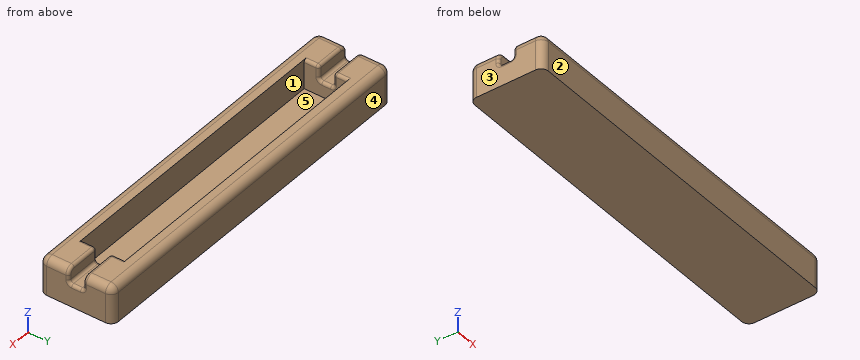
from build123d import *

# Parameters (mm, degrees)
F0_W         = 25
F0_H         = 5
F1_DEPTH     = 2.5
F2_W         = 20
F2_H         = 3
F3_DEPTH     = 2
F4_W         = 2.5
F4_H         = 1
F5_DEPTH     = 1
F6_F1_R      = 0.2
F6_F2_R      = 0.2
F7_T1_DEPTH  = 24
F7_T3_DEPTH  = 1.5
F7_T5_DEPTH  = 3.25
F7_T7_DEPTH  = 1.5
F7_T10_ANGLE = 90
F7_T12_ANGLE = 90
F7_T14_ANGLE = 90
F7_T16_ANGLE = 90
F7_S19_W     = 0.5
F7_S19_H     = 0.5
F7_T20_DEPTH = 0.5
F7_S25_W     = 0.5
F7_S25_H     = 0.5
F7_T26_DEPTH = 0.5
F7_S31_W     = 0.5
F7_S31_H     = 0.5
F7_T32_DEPTH = 0.5
F7_S37_W     = 0.5
F7_S37_H     = 0.5
F7_T38_DEPTH = 0.5


# Not quite as in the source:
# - a fillet or chamfer that OpenCascade refuses, or shapes differently, is made with other operations: its cross-section is extruded or revolved along the edge and cut away or added


with BuildPart() as f1:
    # F0 (on Top) → F1 (new body)
    with BuildSketch(Plane.XY):
        Rectangle(F0_W, F0_H)
    extrude(amount=F1_DEPTH)

    # F2 (on face) → F3 (cut)
    with BuildSketch(Plane.XY.offset(2.5)):
        Rectangle(F2_W, F2_H)
    extrude(amount=-F3_DEPTH, mode=Mode.SUBTRACT)

    # F4 (on face) → F5 (cut)
    with BuildSketch(Plane.XY.offset(2.5)):
        with Locations((-11.25, 0)):
            Rectangle(F4_W, F4_H)
        with Locations((11.25, 0)):
            Rectangle(F4_W, F4_H)
    extrude(amount=-F5_DEPTH, mode=Mode.SUBTRACT)

    # F6: fillet of radius 0.2 on 16 edges, made by hand

    # F6_f1
    f6_f1_edges = [f1.edges().sort_by_distance(p)[0] for p in [
        (-11.25, -0.5, 1.5),
        (-11.25, 0.5, 1.5),
        (11.25, -0.5, 1.5),
        (11.25, 0.5, 1.5),
    ]]
    fillet(f6_f1_edges, radius=F6_F1_R)

    # F6_f2
    f6_f2_edges = [f1.edges().sort_by_distance(p)[0] for p in [
        (-10, -0.5, 2.1),
        (10, 0, 1.5),
        (12.5, -0.5, 2.1),
        (-12.5, 0.5, 2.1),
        (-11.25, 0.5, 2.5),
        (-11.25, -0.5, 2.5),
        (11.25, 0.5, 2.5),
        (11.25, -0.5, 2.5),
        (-10, 1, 2.5),
        (10, 1, 2.5),
        (10, -1, 2.5),
        (-10, -1, 2.5),
        (-12.5, 0.4414213562, 1.5585786438),
        (12.5, -0.4414213562, 1.5585786438),
        (10, 0.4414213562, 1.5585786438),
        (10, -0.4414213562, 1.5585786438),
        (-10, -0.4414213562, 1.5585786438),
    ]]
    fillet(f6_f2_edges, radius=F6_F2_R)

    # F7: fillet of radius 0.5 on 10 edges, made by hand

    # F7_s2 → F7_t1 (cut)
    with BuildSketch(Plane.YZ.offset(-12)):
        with BuildLine():
            ThreePointArc((-2.5, 2), (-2.3535533906, 2.3535533906), (-2, 2.5))
            Line((-2, 2.5), (-2.5, 2.5))
            Line((-2.5, 2.5), (-2.5, 2))
        make_face()
        with BuildLine():
            ThreePointArc((2, 2.5), (2.3535533906, 2.3535533906), (2.5, 2))
            Line((2.5, 2), (2.5, 2.5))
            Line((2.5, 2.5), (2, 2.5))
        make_face()
    extrude(amount=F7_T1_DEPTH, mode=Mode.SUBTRACT)

    # F7_s4 → F7_t3 (cut)
    with BuildSketch(Plane.XZ.offset(0.5)):
        with BuildLine():
            ThreePointArc((-12, 2.5), (-12.3535533906, 2.3535533906), (-12.5, 2))
            Line((-12.5, 2), (-12.5, 2.5))
            Line((-12.5, 2.5), (-12, 2.5))
        make_face()
        with BuildLine():
            ThreePointArc((12.5, 2), (12.3535533906, 2.3535533906), (12, 2.5))
            Line((12, 2.5), (12.5, 2.5))
            Line((12.5, 2.5), (12.5, 2))
        make_face()
    extrude(amount=F7_T3_DEPTH, mode=Mode.SUBTRACT)

    # F7_s6 → F7_t5 (cut)
    with BuildSketch(Plane.XY.offset(-1.25)):
        with BuildLine():
            ThreePointArc((-12, -2.5), (-12.3535533906, -2.3535533906), (-12.5, -2))
            Line((-12.5, -2), (-12.5, -2.5))
            Line((-12.5, -2.5), (-12, -2.5))
        make_face()
        with BuildLine():
            ThreePointArc((12.5, -2), (12.3535533906, -2.3535533906), (12, -2.5))
            Line((12, -2.5), (12.5, -2.5))
            Line((12.5, -2.5), (12.5, -2))
        make_face()
        with BuildLine():
            ThreePointArc((-12, 2.5), (-12.3535533906, 2.3535533906), (-12.5, 2))
            Line((-12.5, 2), (-12.5, 2.5))
            Line((-12.5, 2.5), (-12, 2.5))
        make_face()
        with BuildLine():
            ThreePointArc((12.5, 2), (12.3535533906, 2.3535533906), (12, 2.5))
            Line((12, 2.5), (12.5, 2.5))
            Line((12.5, 2.5), (12.5, 2))
        make_face()
    extrude(amount=F7_T5_DEPTH, mode=Mode.SUBTRACT)

    # F7_s8 → F7_t7 (cut)
    with BuildSketch(Plane.XZ.offset(-2)):
        with BuildLine():
            ThreePointArc((-12, 2.5), (-12.3535533906, 2.3535533906), (-12.5, 2))
            Line((-12.5, 2), (-12.5, 2.5))
            Line((-12.5, 2.5), (-12, 2.5))
        make_face()
        with BuildLine():
            ThreePointArc((12.5, 2), (12.3535533906, 2.3535533906), (12, 2.5))
            Line((12, 2.5), (12.5, 2.5))
            Line((12.5, 2.5), (12.5, 2))
        make_face()
    extrude(amount=F7_T7_DEPTH, mode=Mode.SUBTRACT)

    # F7_s9 → F7_t10 (revolve, cut)
    with BuildSketch(Plane.XY.offset(2)):
        with BuildLine():
            ThreePointArc((12.3, 0.5), (12.4414213562, 0.5585786438), (12.5, 0.7))
            Line((12.5, 0.7), (12.5, 0.5))
            Line((12.5, 0.5), (12.3, 0.5))
        make_face()
    revolve(axis=Axis((12, 0.5, 2), (0, -1, 0)), revolution_arc=F7_T10_ANGLE, mode=Mode.SUBTRACT)

    # F7_s11 → F7_t12 (revolve, cut)
    with BuildSketch(Plane.YZ.offset(-12)):
        with BuildLine():
            ThreePointArc((0.5, 2.3), (0.5585786438, 2.4414213562), (0.7, 2.5))
            Line((0.7, 2.5), (0.5, 2.5))
            Line((0.5, 2.5), (0.5, 2.3))
        make_face()
    revolve(axis=Axis((-12, 0.5, 2), (0, -1, 0)), revolution_arc=F7_T12_ANGLE, mode=Mode.SUBTRACT)

    # F7_s13 → F7_t14 (revolve, cut)
    with BuildSketch(Plane.YZ.offset(12)):
        with BuildLine():
            ThreePointArc((-0.5, 2.3), (-0.5585786438, 2.4414213562), (-0.7, 2.5))
            Line((-0.7, 2.5), (-0.5, 2.5))
            Line((-0.5, 2.5), (-0.5, 2.3))
        make_face()
    revolve(axis=Axis((12, -0.5, 2), (0, 1, 0)), revolution_arc=F7_T14_ANGLE, mode=Mode.SUBTRACT)

    # F7_s15 → F7_t16 (revolve, cut)
    with BuildSketch(Plane.XY.offset(2)):
        with BuildLine():
            ThreePointArc((-12.3, -0.5), (-12.4414213562, -0.5585786438), (-12.5, -0.7))
            Line((-12.5, -0.7), (-12.5, -0.5))
            Line((-12.5, -0.5), (-12.3, -0.5))
        make_face()
    revolve(axis=Axis((-12, -0.5, 2), (0, 1, 0)), revolution_arc=F7_T16_ANGLE, mode=Mode.SUBTRACT)


with BuildPart() as f7_tool18:
    # F7_s19 → F7_t20 (new body)
    with BuildSketch(Plane.XY.offset(2)):
        with Locations((-12.25, -2.25)):
            Rectangle(F7_S19_W, F7_S19_H)
    extrude(amount=F7_T20_DEPTH)

    # F7_s21 → F7_t22 (revolve, cut)
    with BuildSketch(Plane(origin=(-12, -2, 2), x_dir=(0.7071067812, 0.7071067812, 0), z_dir=(0.7071067812, -0.7071067812, 0))):
        with BuildLine():
            ThreePointArc((0, -0.5), (0.5, 0), (0, 0.5))
            Line((0, 0.5), (0, -0.5))
        make_face()
    revolve(axis=Axis((-12, -2, 2), (0, 0, 1)), mode=Mode.SUBTRACT)


with BuildPart() as f1_1:
    add(f1.part)

    # F7_t17: cut F7_tool18
    add(f7_tool18.part, mode=Mode.SUBTRACT)


with BuildPart() as f7_tool24:
    # F7_s25 → F7_t26 (new body)
    with BuildSketch(Plane.YZ.offset(12)):
        with Locations((-2.25, 2.25)):
            Rectangle(F7_S25_W, F7_S25_H)
    extrude(amount=F7_T26_DEPTH)

    # F7_s27 → F7_t28 (revolve, cut)
    with BuildSketch(Plane(origin=(12, -2, 2), x_dir=(0, 0.7071067812, -0.7071067812), z_dir=(0, -0.7071067812, -0.7071067812))):
        with BuildLine():
            ThreePointArc((0, -0.5), (0.5, 0), (0, 0.5))
            Line((0, 0.5), (0, -0.5))
        make_face()
    revolve(axis=Axis((12, -2, 2), (1, 0, 0)), mode=Mode.SUBTRACT)


with BuildPart() as f1_2:
    add(f1_1.part)

    # F7_t23: cut F7_tool24
    add(f7_tool24.part, mode=Mode.SUBTRACT)


with BuildPart() as f7_tool30:
    # F7_s31 → F7_t32 (new body)
    with BuildSketch(Plane.YZ.offset(12)):
        with Locations((2.25, 2.25)):
            Rectangle(F7_S31_W, F7_S31_H)
    extrude(amount=F7_T32_DEPTH)

    # F7_s33 → F7_t34 (revolve, cut)
    with BuildSketch(Plane(origin=(12, 2, 2), x_dir=(0, -0.7071067812, -0.7071067812), z_dir=(0, -0.7071067812, 0.7071067812))):
        with BuildLine():
            ThreePointArc((0, -0.5), (0.5, 0), (0, 0.5))
            Line((0, 0.5), (0, -0.5))
        make_face()
    revolve(axis=Axis((12, 2, 2), (1, 0, 0)), mode=Mode.SUBTRACT)


with BuildPart() as f1_3:
    add(f1_2.part)

    # F7_t29: cut F7_tool30
    add(f7_tool30.part, mode=Mode.SUBTRACT)


with BuildPart() as f7_tool36:
    # F7_s37 → F7_t38 (new body)
    with BuildSketch(Plane.YZ.offset(-12)):
        with Locations((2.25, 2.25)):
            Rectangle(F7_S37_W, F7_S37_H)
    extrude(amount=-F7_T38_DEPTH)

    # F7_s39 → F7_t40 (revolve, cut)
    with BuildSketch(Plane(origin=(-12, 2, 2), x_dir=(0, -0.7071067812, -0.7071067812), z_dir=(0, 0.7071067812, -0.7071067812))):
        with BuildLine():
            ThreePointArc((0, -0.5), (0.5, 0), (0, 0.5))
            Line((0, 0.5), (0, -0.5))
        make_face()
    revolve(axis=Axis((-12, 2, 2), (-1, 0, 0)), mode=Mode.SUBTRACT)


with BuildPart() as f1_4:
    add(f1_3.part)

    # F7_t35: cut F7_tool36
    add(f7_tool36.part, mode=Mode.SUBTRACT)


solid = f1_4.part
Source: CAD feature listing. Evaluate the final solid. Frame: model axes, mm. Face numbers are marked on the shaded views. A direction names the side the tool comes from. Give positions to 0.01 mm unless a question says otherwise; leave off trailing zeros. Loops run counter-clockwise (first coordinate to the right, second up) from the corner with the lowest first, then second, coordinate; pieces in that order, holes last. Notation, with made-up numbers: (-12.75, 17.25) -> (22.25, 17.25) arc R29 ccw to (22.25, 48.25) -> close; hole circle Ø7 at (30.25, -0.75). An arc over 180 degrees is marked (long way). Use a Markdown table: item, result. Add a question column.
1) Line query: line 1 along X through (y, z) = (0.75, 1); line 2 along Y through (x, z) = (-1.75, 0.55); line 3 along Y through (x, z) = (10.25, 1.9). Output: solid intervals per line, ascending. Write a range as [from, to].
2) First-contact query: pin 1 (0.5 mm diameter, centred on x = 11.5, y = 0, fed in from +Z); pin 2 (0.9 mm diameter, centred on x = 1.5, y = -0.5, fed in from +Z). Flat tips, straight axial feed; report the tip coordinate or a pass-through.
3) Section query B-B, the plane x = 6.75. Return the cut outline in (y, z), then the cut area to 3 significant figures.
4) Reachability of the marked faces 1 and 2 from +Z, -Z, +X, -X, +Y, -Y: full face, straight path, thin tool, end or side. Return the list, or none.
5) Section query C-C, the plane z = 0.9. Return the cut outline in (x, y), then the cut area to 3 significant figures.
6) Pull-direction query (X, two-part tool) for the marked faces 3, 4 and 5; classes: +X half, -X half, draft (parallel to the pull), parting line (faces both ways), or undercut.
7) Section query A-A, the plane y = -1.05. Return the cut outline in (x, z), then the cut area to 3 significant figures.
Numbers:
| question | item | result |
|---|---|---|
| 1 | line 1 | x = [-12.5, -10], [10, 12.5] |
| 1 | line 2 | y = [-2.5, -1.5], [1.5, 2.5] |
| 1 | line 3 | y = [-2.5, -0.5], [0.5, 2.5] |
| 2 | pin 1 | stops at z = 1.5 |
| 2 | pin 2 | stops at z = 0.5 |
| 3 | outline | (-2.5, 0) -> (2.5, 0) -> (2.5, 2) arc R0.5 ccw to (2, 2.5) -> (1.5, 2.5) -> (1.5, 0.5) -> (-1.5, 0.5) -> (-1.5, 2.5) -> (-2, 2.5) arc R0.5 ccw to (-2.5, 2) -> close |
| 3 | area | 6.39 mm2 |
| 4 | face 1 | +Z |
| 4 | face 2 | +Z, -Z, +X, -X, -Y |
| 5 | outline | (-12.5, -2) arc R0.5 ccw to (-12, -2.5) -> (12, -2.5) arc R0.5 ccw to (12.5, -2) -> (12.5, 2) arc R0.5 ccw to (12, 2.5) -> (-12, 2.5) arc R0.5 ccw to (-12.5, 2) -> close; hole (-10, -1.5) -> (10, -1.5) -> (10, 1.5) -> (-10, 1.5) -> close |
| 5 | area | 64.8 mm2 |
| 6 | face 3 | -X half |
| 6 | face 4 | draft |
| 6 | face 5 | undercut |
| 7 | outline | (-12.5, 0) -> (12.5, 0) -> (12.5, 2) arc R0.5 ccw to (12, 2.5) -> (10.2, 2.5) arc R0.2 ccw to (10, 2.3) -> (10, 0.5) -> (-10, 0.5) -> (-10, 2.3) arc R0.2 ccw to (-10.2, 2.5) -> (-12, 2.5) arc R0.5 ccw to (-12.5, 2) -> close |
| 7 | area | 22.4 mm2 |
